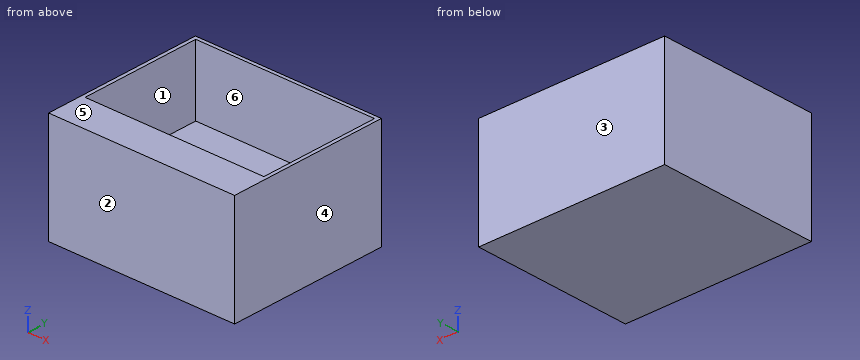
from build123d import *

# Parameters (mm, degrees)
F0_W     = 132.037088275
F0_H     = 113.3796721697
F1_DEPTH = 76.708
F2_T     = -2.54
F3_DEPTH = 25.4
F4_DEPTH = 25.4


with BuildPart() as f1:
    # F0 (on Top) → F1 (new body)
    with BuildSketch(Plane.XY):
        Rectangle(F0_W, F0_H)
    extrude(amount=F1_DEPTH)

    # F2
    f2_openings = [f1.faces().sort_by_distance(p)[0] for p in [
        (0, 0, 76.708),
    ]]
    offset(amount=F2_T, openings=f2_openings)

    # F3 (add): a face of the model
    f3_faces = [f1.faces().sort_by_distance(p)[0] for p in [
        (0, 0, 2.54),
    ]]
    extrude(f3_faces, amount=F3_DEPTH)

    # F4 (add): a face of the model
    f4_faces = [f1.faces().sort_by_distance(p)[0] for p in [
        (0, -56.6898360848, 38.354),
    ]]
    extrude(f4_faces, amount=-F4_DEPTH)


solid = f1.part
Work out the finished part from the listing and answer in its coordinate system (mm). Face numbers are marked on the shaded views. A direction names the side the tool comes from. Round coordinates to 2 decimals unless told otherwise and drop trailing zeros. Order: outer loops, then holes, each group sorted by start corner. A loop starts at its lowest first (then second) coordinate and runs counter-clockwise, first axis right, second up. Notation, with made-up numbers: M 7,-2.5 L 35,-2.5 A22 cw 35,23.5 Z; hole C 42.25,67.5 d2. An arc over 180 degrees is marked long. One line per item, written item: value.
Q1. Flat-ended cylindrical pins translate along their axes: pin 1 (2 mm diameter, centred on x = -48.5, y = -12, fed in from -Z); pin 2 (1 mm diameter, centred on x = 47.5, y = 6, fed in from +Z). Find the tip coordinate at first contact, or state that the pin passes through.
Derived:
pin 1: z = 0
pin 2: z = 27.94
Q2. Determine the mould class of the marked faces 1, 2, 3 and 4 for opening direction Y: released by +Y, released by -Y, zero draft, split by the parting line, or undercut.
Derived:
face 1: undercut
face 2: released by -Y
face 3: released by +Y
face 4: zero draft
Q3. For the marked faces 5 and 6, determine the directions among +Z, -Z, +X, -X, +Y, -Y from which every point of the face is accessible in a straight line to the end or side of a thin tool.
Derived:
face 5: +Z, +X, -X, +Y, -Y
face 6: +Z
Q4. Find section B-B on y = -18. Write down the section's boundary in (x, z).
Derived:
outline: M -66.02,0 L 66.02,0 L 66.02,76.71 L 63.48,76.71 L 63.48,27.94 L -63.48,27.94 L -63.48,76.71 L -66.02,76.71 Z
Q5. Straight lines are drawn through the part: line 1 (X direction, y = 37, z = 70); line 2 (Y direction, x = -45.5, z = 51); line 3 (Z direction, x = -36.5, y = 52). For each, find the intervals that lie inside material, in ascending order.
Derived:
line 1: -66.02 to -63.48, 63.48 to 66.02
line 2: -56.69 to -31.29, 54.15 to 56.69
line 3: 0 to 27.94
Q6. Find section A-A on z = 60. Write down the section's boundary in (x, y).
Derived:
outline: M -66.02,-56.69 L 66.02,-56.69 L 66.02,56.69 L -66.02,56.69 Z; hole M -63.48,-31.29 L 63.48,-31.29 L 63.48,54.15 L -63.48,54.15 Z
Q7. Find section C-C on x = 3. Write down the section's boundary in (y, z).
Derived:
outline: M -56.69,0 L 56.69,0 L 56.69,76.71 L 54.15,76.71 L 54.15,27.94 L -31.29,27.94 L -31.29,76.71 L -56.69,76.71 Z
